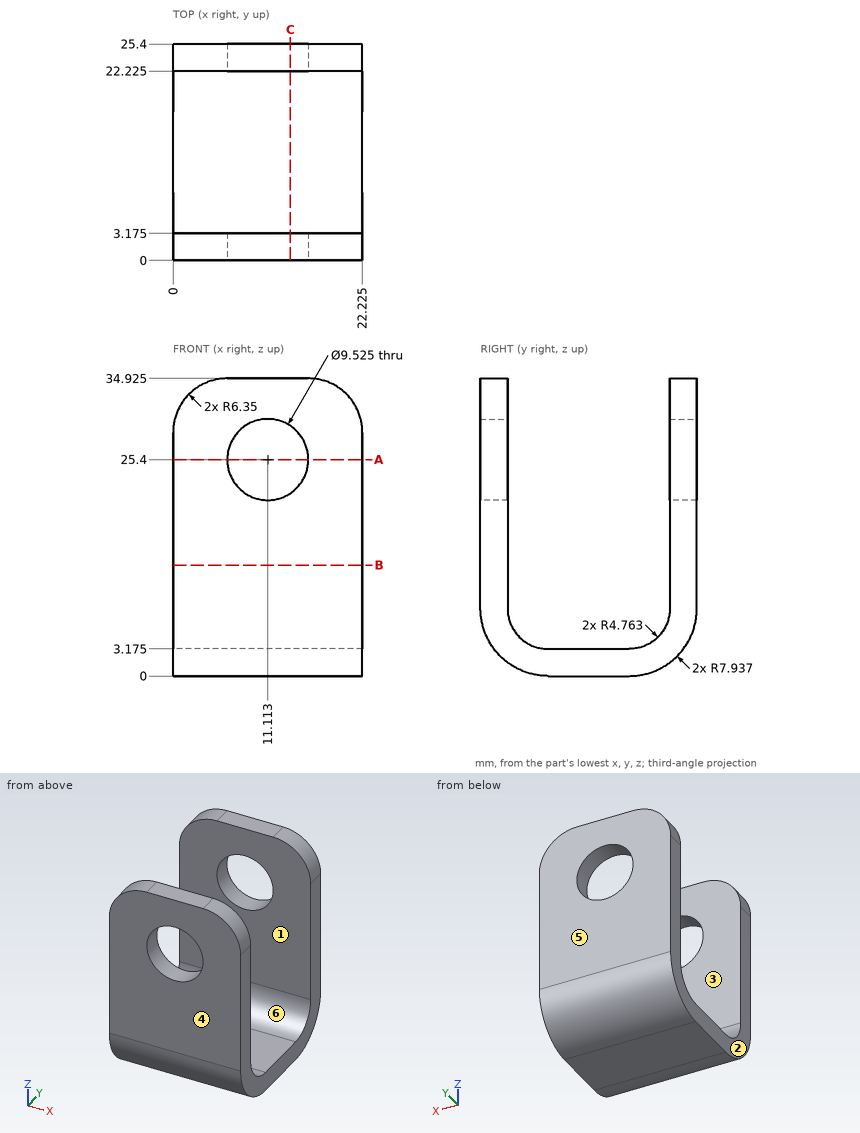
Here's the drawing with two shaded views (mm, measured from the low corner). I have some questions. A direction names the side the tool comes from. Give positions to 0.01 mm unless a question says otherwise; leave off trailing zeros. Write each loop counter-clockwise with the first axis right and the second up, starting at its lowest first coordinate (ties: lowest second). Pieces come first, ordered by that corner, then holes. Notation, with made-up numbers: (-16, -4.5) - (17, -4.5) arc R28 cw to (17, 17.5) - close; hole circle Ø10 at (46, 15). An arc over 180 degrees is marked (long way). One line per item, written item: value. Start each with the question number.
Item 1: Imagine slicing it at A-A, the plane z = 25.4. Give the number of separate pieces and of enclosed holes in the cut face.
Item 2: If we mould it in two halves opening along Y, with no side actions, what happens to the marked faces 3, 4, 5 and 6? For each: +Y half, -Y half, draft (parallel to the pull), parting line (faces both ways), or undercut.
Item 3: Which directions (+Z, -Z, +X, -X, +Y, -Y) give clear straight access to the entire face, cutting with the end or side of a thin tool? Please do the marked faces 1 and 2.
Item 4: I'm going to push flat-ended pins straight in: pin 1 (1 mm diameter, centred on x = 7, y = 6.5, fed in from +Z); pin 2 (8 mm diameter, centred on x = 3.5, y = 4.5, fed in from -Z); pin 3 (3 mm diameter, centred on x = 3.5, y = 2.5, fed in from -Z) (1 decimal); pin 4 (4 mm diameter, centred on x = 6.5, y = 10.5, fed in from +Z) (1 decimal). Where does each tip first touch, or does it pass through?
Item 5: Imagine slicing it at C-C, the plane x = 13.75. List the corners of the cut face in (y, z) for me (1 decimal).
Item 6: Please list where these lines run through material, in increasing order: line 1 (Y direction, x = 15.25, z = 20.5) (1 decimal); line 2 (Z direction, x = 17.5, y = 10.75) (1 decimal); line 3 (Y direction, x = 18, z = 5) (1 decimal). Write a range as from..to.
Item 7: Imagine slicing it at B-B, the plane z = 13. List the corners of the cut face in (x, y) for me (1 decimal).
Geometry says:
1. separate pieces: 4
1. enclosed holes: 0
2. face 3: undercut
2. face 4: -Y half
2. face 5: +Y half
2. face 6: undercut
3. face 1: +Z, +X, -X
3. face 2: +Z, -Z, -X, +Y, -Y
4. pin 1: z = 3.59
4. pin 2: z = 0
4. pin 3: z = 1
4. pin 4: z = 3.2
5. outline: (0, 7.9) arc R7.9 ccw to (7.9, 0) - (17.5, 0) arc R7.9 ccw to (25.4, 7.9) - (25.4, 21.4) - (22.2, 21.4) - (22.2, 7.9) arc R4.8 cw to (17.5, 3.2) - (7.9, 3.2) arc R4.8 cw to (3.2, 7.9) - (3.2, 21.4) - (0, 21.4) - close; (0, 29.4) - (3.2, 29.4) - (3.2, 34.9) - (0, 34.9) - close; (22.2, 29.4) - (25.4, 29.4) - (25.4, 34.9) - (22.2, 34.9) - close
6. line 1: 0..3.2, 22.2..25.4
6. line 2: 0..3.2
6. line 3: 0.6..4.2, 21.2..24.8
7. outline: (0, 0) - (22.2, 0) - (22.2, 3.2) - (0, 3.2) - close; (0, 22.2) - (22.2, 22.2) - (22.2, 25.4) - (0, 25.4) - close
